For this review, use the dimensioned drawing (mm, ordinates from the lowest corner) and the shaded views. A direction names the side the tool comes from. Round coordinates to 2 decimals unless told otherwise and drop trailing zeros. Loops run counter-clockwise (first coordinate to the right, second up) from the corner with the lowest first, then second, coordinate; pieces in that order, holes last.
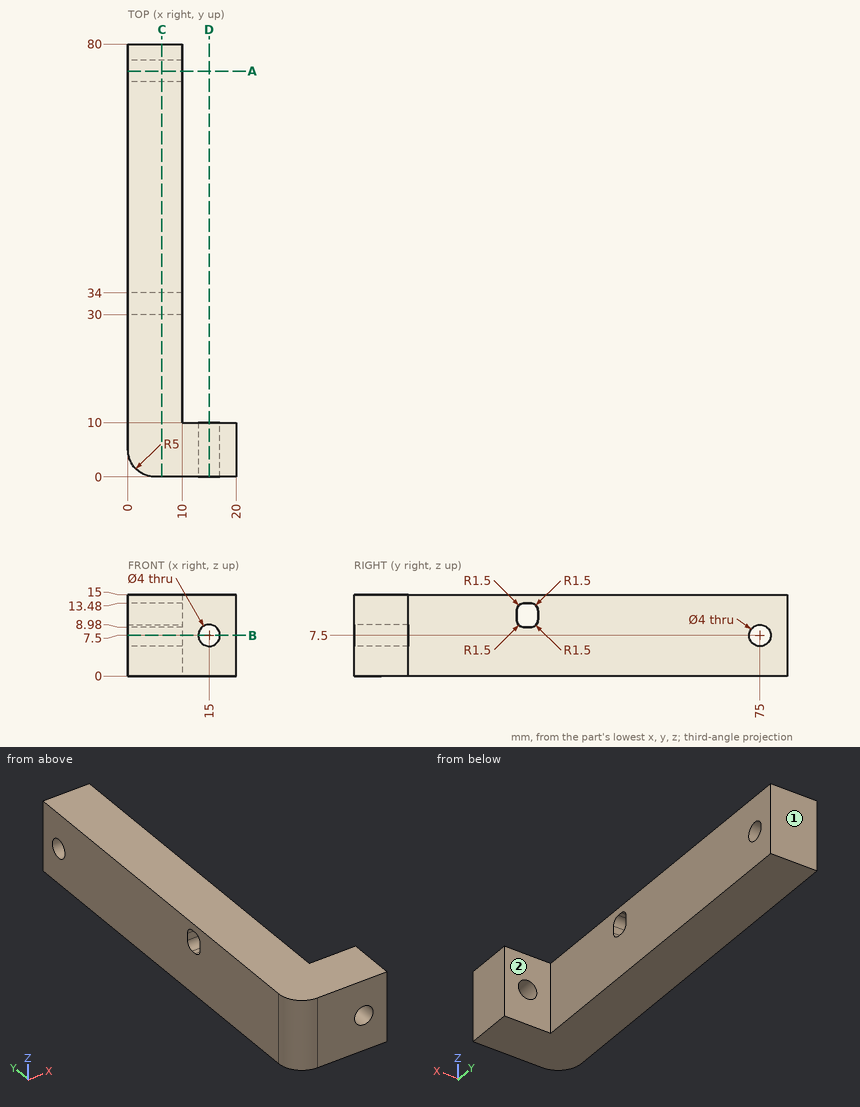
(1) For L1, parallel to Z at x = 15, y = 3.75; L2, parallel to Y at x = 7.5, z = 7.5; L3, parallel to X at y = 60, z = 9.75, list the stretches that pass through material, from the lowest coordinate up.
(2) For the marked faces 1 and 2, list the 3-axis set-ups (+Z, -Z, +X, -X, +Y, -Y) from which the entire face can be reached by the end or side of a thin tool; tool diameter is ignored.
(3) Insertion check: pin 1 Ø2 at (y, z) = (68.5, 8.5) entering from +X; pin 2 Ø1.2 at (x, z) = (3, 11.5) entering from -Y. Each pin has a flat end and moves straight along its axis. Give the tip position at first contact, or say it passes through.
(4) Add section A-A (y = 75). Give the boundary of the cut face in (x, z).
(5) Add section C-C (x = 6.25). Give the boundary of the cut face in (y, z), plus the area to 3 significant figures.
(6) Add section B-B (z = 7.5). Give the boundary of the cut face in (x, y).
Outcome:
1. L1: z = 0 to 5.5, 9.5 to 15
1. L2: y = 0 to 73, 77 to 80
1. L3: x = 0 to 10
2. face 1: +Z, -Z, +X, -X, +Y
2. face 2: +Z, -Z, +X, +Y
3. pin 1: stops at x = 10
3. pin 2: stops at y = 0.2
4. outline: (0, 0) - (10, 0) - (10, 5.5) - (0, 5.5) - close; (0, 9.5) - (10, 9.5) - (10, 15) - (0, 15) - close
5. outline: (0, 0) - (80, 0) - (80, 15) - (0, 15) - close; hole (30, 10.48) arc R1.5 ccw to (31.5, 8.98) - (32.5, 8.98) arc R1.5 ccw to (34, 10.48) - (34, 11.98) arc R1.5 ccw to (32.5, 13.48) - (31.5, 13.48) arc R1.5 ccw to (30, 11.98) - close; hole circle Ø4 at (75, 7.5)
5. area: 1,170 mm2
6. outline: (0, 5) arc R5 ccw to (5, 0) - (13, 0) - (13, 10) - (10, 10) - (10, 73) - (0, 73) - close; (0, 77) - (10, 77) - (10, 80) - (0, 80) - close; (17, 0) - (20, 0) - (20, 10) - (17, 10) - close
